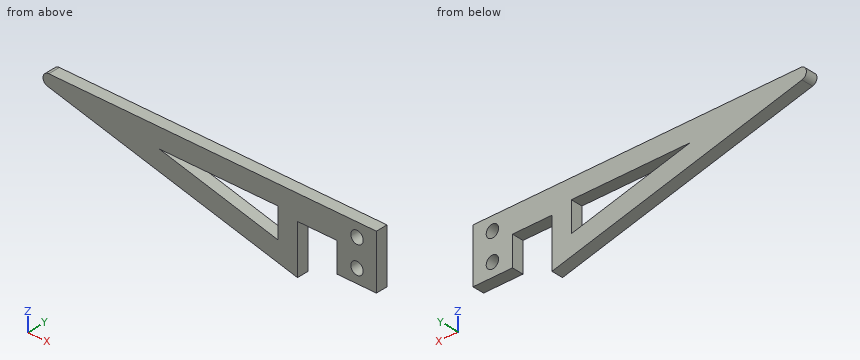
from build123d import *

# Parameters (mm, degrees)
SKETCH2_R           = 1.6
BOSS_EXTRUDE1_DEPTH = 3.0226
FILLET1_R           = 1.5


with BuildPart() as part:
    # Sketch2 → Boss-Extrude1 (new body)
    with BuildSketch(Plane(origin=(0, 0, 0), x_dir=(1, 0, 0), z_dir=(0, 1, 0))):
        Polygon((0, -6.35), (-96.5, -6.35), (-20.32, 12.73), (-20.32, 0.03), (-10.16, 0.03), (-10.16, 7.65), (0, 7.65), align=None)
        with Locations(Location((-5, -2.85, 0), (0, 0, 270))):
            Circle(SKETCH2_R, mode=Mode.SUBTRACT)
        with Locations(Location((-5, 4.15, 0), (0, 0, 270))):
            Circle(SKETCH2_R, mode=Mode.SUBTRACT)
        Polygon((-25.32, -1.35), (-25.32, 6.323263145), (-55.956749809, -1.35), align=None, mode=Mode.SUBTRACT)
    extrude(amount=BOSS_EXTRUDE1_DEPTH)

    # Fillet1
    fillet1_edges = [part.edges().sort_by_distance(p)[0] for p in [
        (-96.5, 1.5113, 6.35),
    ]]
    fillet(fillet1_edges, radius=FILLET1_R)


solid = part.part
Source: CAD feature listing. Evaluate the final solid. Frame: model axes, mm. Round coordinates to 2 decimals unless told otherwise and drop trailing zeros. Write each loop counter-clockwise with the first axis right and the second up, starting at its lowest first coordinate (ties: lowest second). Pieces come first, ordered by that corner, then holes. Notation, with made-up numbers: (12.25, 70) - (66.25, 70) arc R21 ccw to (66.25, 88) - close; hole circle Ø2 at (58, -18.75). An arc over 180 degrees is marked (long way). Use CSV: the item, a comma, the result in double quotes. Start each with the question number.
(1) First-contact query: pin 1 Ø3.5 at (x, z) = (-5, -4.15) entering from -Y; pin 2 Ø0.9 at (x, y) = (-4.5, 1.5) entering from -Z. Flat tips, straight axial feed; report the tip coordinate or a pass-through.
(2) Cut plane B-B, the plane y = 1.8. Return loops of the section in (x, z).
(3) Cut plane D-D, the plane x = -45.5. Return loops of the section in (y, z).
(4) Material intervals for probe 1 along Z at (x, y) = (-17, 0.55); probe 2 along Z at (x, y) = (-52.5, 0.3); probe 3 along Z at (x, y) = (-22.5, 0.3), sorted ascending. Write a range as [from, to].
(5) Cut plane A-A, the plane x = -5. Return loops of the section in (y, z), and give its area (3 significant figures).
(6) Cut plane C-C, the plane z = -1. Return loops of the section in (x, y).
Geometry says:
1,pin 1,"y = 0"
1,pin 2,"z = -7.65"
2,outline,"(-84.7, 3.39) - (-20.32, -12.73) - (-20.32, -0.03) - (-10.16, -0.03) - (-10.16, -7.65) - (0, -7.65) - (0, 6.35) - (-84.34, 6.35) arc R1.5 ccw to start; hole (-55.96, 1.35) - (-25.32, -6.32) - (-25.32, 1.35) - close; hole circle Ø3.2 at (-5, -4.15); hole circle Ø3.2 at (-5, 2.85)"
3,outline,"(0, -6.42) - (3.02, -6.42) - (3.02, -1.27) - (0, -1.27) - close; (0, 1.35) - (3.02, 1.35) - (3.02, 6.35) - (0, 6.35) - close"
4,probe 1,"[-0.03, 6.35]"
4,probe 2,"[-4.67, 0.48], [1.35, 6.35]"
4,probe 3,"[-12.18, 6.35]"
5,outline,"(0, -7.65) - (3.02, -7.65) - (3.02, -5.75) - (0, -5.75) - close; (0, -2.55) - (3.02, -2.55) - (3.02, 1.25) - (0, 1.25) - close; (0, 4.45) - (3.02, 4.45) - (3.02, 6.35) - (0, 6.35) - close"
5,area,"23.0 mm²"
6,outline,"(-67.15, 0) - (-46.57, 0) - (-46.57, 3.02) - (-67.15, 3.02) - close; (-25.32, 0) - (-20.32, 0) - (-20.32, 3.02) - (-25.32, 3.02) - close; (-10.16, 0) - (0, 0) - (0, 3.02) - (-10.16, 3.02) - close"
